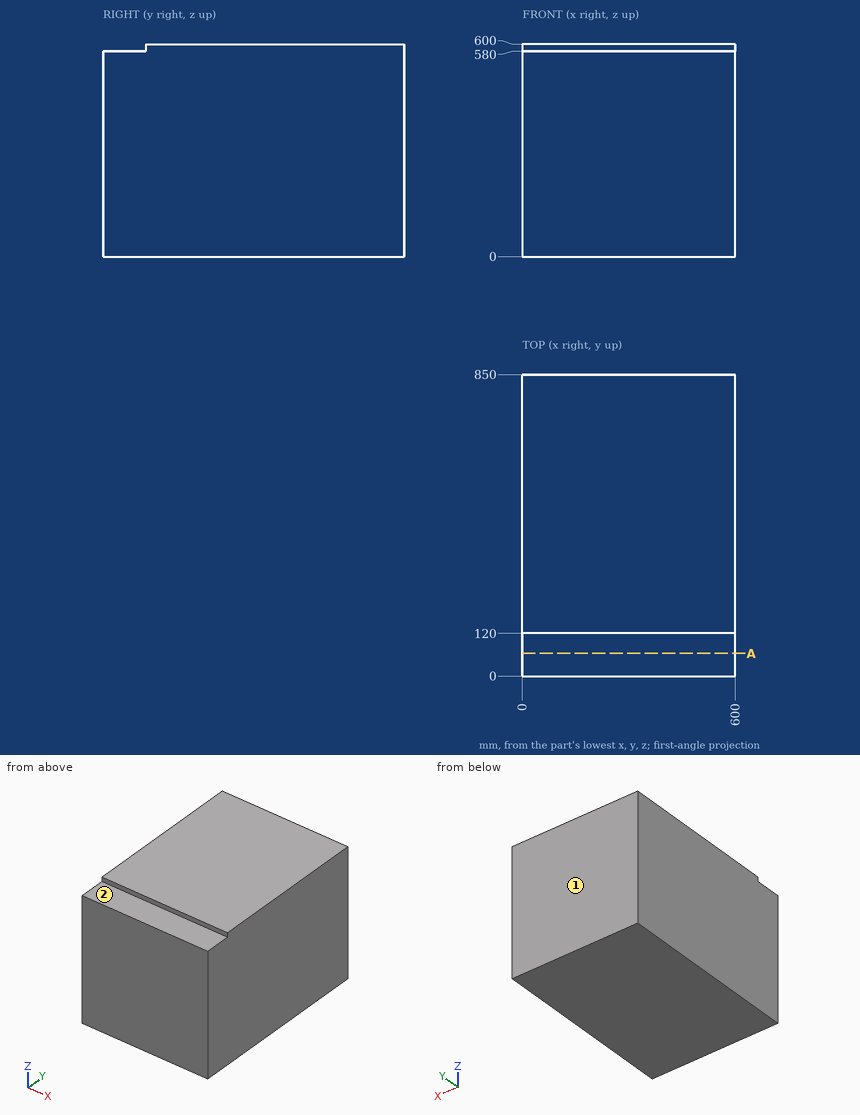
Study the drawing (mm; zero at the part's minimum x, y, z) and answer. A direction names the side the tool comes from. Coordinates: 2 decimals unless noted, no trailing zeros. Write each loop counter-clockwise with the first axis right and the second up, starting at its lowest first coordinate (ties: lowest second). Pieces come first, ordered by that corner, then holes. Notation, with made-up numbers: M 14.25,66 L 57.25,66 A28 cw 57.25,98 Z; hole C 24.5,-38 d3. An arc over 180 degrees is marked long. Use a Markdown table: item, result. Add a question column.
1. Which of the six approach directions +Z, -Z, +X, -X, +Y, -Y give full straight-line access (tool end or side, diameter ignored) to the marked faces 1 and 2?
2. Section A-A (y = 64) is taken. Give the vertices of the cut face in (x, z), plus the area to 3 significant figures.
3. A straight line is drawn through the part: line 1 along Z through (x, y) = (47.5, 48.5). Find the intervals that lie inside material, in ascending order. Write a range as [from, to].
Data:
| question | item | result |
|---|---|---|
| 1 | face 1 | +Z, -Z, +X, -X, +Y |
| 1 | face 2 | +Z, +X, -X, -Y |
| 2 | outline | M 0,0 L 600,0 L 600,580 L 0,580 Z |
| 2 | area | 348,000 mm2 |
| 3 | line 1 | z = [0, 580] |
